Check sheet for the modelled part. Datum: model origin and axes. Units: mm. A direction names the side the tool comes from. Coordinates: 2 decimals unless noted, no trailing zeros. Loops run counter-clockwise (first coordinate to the right, second up) from the corner with the lowest first, then second, coordinate; pieces in that order, holes last. Notation, with made-up numbers: (68, 56) - (77, 56) arc R15 cw to (77, 60) - close; hole circle Ø5 at (86, -19.5). An arc over 180 degrees is marked (long way). Use a Markdown table: item, result. Add a question column.
1) Go/stop test with flat-tipped pins: P1, Ø3, axis at x = -3, y = 2.5, coming from the +Z side; P2, Ø2, axis at x = -2, y = 2, coming from the -Z side (3 decimals); P3, Ø3, axis at x = 4.5, y = -1, coming from the +Z side. Record where each tip stops, or that it passes through.
2) Sectioned sample at C-C, the plane y = 1.5. Enter the section's corners in (x, z) (3 decimals), then the cut area to 4 significant figures.
3) Sectioned sample at B-B, the plane z = -11. Enter the section's corners in (x, y) (3 decimals), then the cut area to 4 significant figures.
4) Tool access check on faces 1 (the cylindrical face through (0.7, 5.76, -45.82)), 2 (the flat face through (0, 2, -12.5)), 3 (the flat face through (0, 4.15, -36)). Record the directions out of +Z, -Z, +X, -X, +Y, -Y that give a thin tool (end or side, any length) a straight path to the whole face; none if there is none.
5) Sectioned sample at A-A, the plane y = 6.5. Enter the section's corners in (x, z) (3 decimals).
6) Draft check along X on faces 4 (the cylindrical face through (-0.348, 6.149, -13.615)), 5 (the cylindrical face through (-3.905, -1.565, -0.867)), 6 (the cylindrical face through (4.946, -1.565, 4.289)). Enter one of: pulls with the +X half, pulls with the -X half, needs draft (parallel to the pull), parting line crosses it, or undercut.
7) Thickness scan on line 1 (Y direction, x = 1, z = -17.5) (3 decimals); line 2 (Z direction, x = -1.5, y = 2.5) (3 decimals); line 3 (Z direction, x = 0.5, y = 7). Record the ranges inside material, lowest first.
from build123d import *

# Parameters (mm, degrees)
SKETCH1_R                    = 4
BASE_FLANGE1_DEPTH           = 3.175
EDGE_FLANGE1_STRIP_W         = 14.1732
EDGE_FLANGE1_STRIP_H         = 3.175
EDGE_FLANGE1_STRIP_CUT_DEPTH = 14
EDGE_FLANGE1_DEPTH           = 14
EDGE_FLANGE2_STRIP_W         = 14.1732
EDGE_FLANGE2_STRIP_H         = 3.175
EDGE_FLANGE2_STRIP_CUT_DEPTH = 14
EDGE_FLANGE2_DEPTH           = 14
SKETCH17_R                   = 3.175
CUT_EXTRUDE1_DEPTH           = 3.175


# Sheet-metal steps are written as plain solids
with BuildPart() as part:
    # Sketch1 → Base-Flange1 (new body)
    with BuildSketch(Plane(origin=(0, 0, 0), x_dir=(1, 0, 0), z_dir=(0, 1, 0))):
        with BuildLine():
            Line((6.750002463, 0), (6.750002463, 12.5))
            Line((6.750002463, 12.5), (-7.249997537, 12.5))
            Line((-7.249997537, 12.5), (-7.249997537, 0))
            ThreePointArc((-7.249997537, 0), (-5.492638224, -4.242640687), (-1.249997537, -6))
            Line((-1.249997537, -6), (0.750002463, -6))
            ThreePointArc((0.750002463, -6), (4.99264315, -4.242640687), (6.750002463, 0))
        make_face()
        with Locations(Location((0, 0, 0), (0, 0, 270))):
            Circle(SKETCH1_R, mode=Mode.SUBTRACT)
    extrude(amount=-BASE_FLANGE1_DEPTH)

    # Edge-Flange1 strip (across the edge) → Edge-Flange1 strip cut (cut)
    with BuildSketch(Plane(origin=(6.750002463, 0, -12.5), x_dir=(0, 0, 1), z_dir=(-1, 0, 0))):
        with Locations((-6.35, -1.5875)):
            Rectangle(EDGE_FLANGE1_STRIP_W, EDGE_FLANGE1_STRIP_H)
    extrude(amount=EDGE_FLANGE1_STRIP_CUT_DEPTH, mode=Mode.SUBTRACT)

    # Edge-Flange1 section (across the edge) → Edge-Flange1 (add)
    with BuildSketch(Plane(origin=(6.750002463, 0, -12.5), x_dir=(0, 0, 1), z_dir=(-1, 0, 0))):
        with BuildLine():
            Line((-3.175, 0.7366), (-3.175, 7.324994814))
            Line((-3.175, 7.324994814), (0, 7.324994814))
            Line((0, 7.324994814), (0, 0.7366))
            ThreePointArc((0, 0.7366), (0.215745145, 0.215745145), (0.7366, 0))
            Line((0.7366, 0), (0.7366, -3.175))
            ThreePointArc((0.7366, -3.175), (-2.029318885, -2.029318885), (-3.175, 0.7366))
        make_face()
    extrude(amount=EDGE_FLANGE1_DEPTH)

    # Edge-Flange2 strip (across the edge) → Edge-Flange2 strip cut (cut)
    with BuildSketch(Plane(origin=(-7.249997537, 7.324994814, -15.675), x_dir=(0, -1, 0), z_dir=(1, 0, 0))):
        with Locations((-3.175, -1.5875)):
            Rectangle(EDGE_FLANGE2_STRIP_W, EDGE_FLANGE2_STRIP_H)
    extrude(amount=EDGE_FLANGE2_STRIP_CUT_DEPTH, mode=Mode.SUBTRACT)

    # Edge-Flange2 section (across the edge) → Edge-Flange2 (add)
    with BuildSketch(Plane(origin=(-7.249997537, 7.324994814, -15.675), x_dir=(0, -1, 0), z_dir=(1, 0, 0))):
        with BuildLine():
            Line((0, 0.7366), (0, 40.175004419))
            Line((0, 40.175004419), (3.175, 40.175004419))
            Line((3.175, 40.175004419), (3.175, 0.7366))
            ThreePointArc((3.175, 0.7366), (3.390745145, 0.215745145), (3.9116, 0))
            Line((3.9116, 0), (3.9116, -3.175))
            ThreePointArc((3.9116, -3.175), (1.145681115, -2.029318885), (0, 0.7366))
        make_face()
    extrude(amount=EDGE_FLANGE2_DEPTH)

    # Sketch17 → Cut-Extrude1 (cut)
    with BuildSketch(Plane(origin=(0, 7.324994814, 0), x_dir=(1, 0, 0), z_dir=(0, 1, 0))):
        with BuildLine():
            ThreePointArc((-7.249997537, 48.850004419), (-5.199745006, 53.799751887), (-0.249997537, 55.850004419))
            Line((-0.249997537, 55.850004419), (-7.249997537, 55.850004419))
            Line((-7.249997537, 55.850004419), (-7.249997537, 48.850004419))
        make_face()
        with BuildLine():
            ThreePointArc((-0.249997537, 55.850004419), (4.699749931, 53.799751887), (6.750002463, 48.850004419))
            Line((6.750002463, 48.850004419), (6.750002463, 55.850004419))
            Line((6.750002463, 55.850004419), (-0.249997537, 55.850004419))
        make_face()
        with Locations(Location((-0.249997537, 48.850004419, 0), (0, 0, 270))):
            Circle(SKETCH17_R)
    extrude(amount=-CUT_EXTRUDE1_DEPTH, mode=Mode.SUBTRACT)


solid = part.part
Solved:
| question | item | result |
|---|---|---|
| 1 | P1 | stops at z = -12.5 |
| 1 | P2 | stops at z = -15.675 |
| 1 | P3 | stops at z = 5.56 |
| 2 | outline | (-7.25, -15.675) - (6.75, -15.675) - (6.75, -12.5) - (-7.25, -12.5) - close |
| 2 | area | 44.45 mm2 |
| 3 | outline | (-7.25, -3.175) - (6.75, -3.175) - (6.75, 0) - (-7.25, 0) - close |
| 3 | area | 44.45 mm2 |
| 4 | face 1 | +Y, -Y |
| 4 | face 2 | +Z, +X, -X, +Y |
| 4 | face 3 | -Z, +X, -X, -Y |
| 5 | outline | (-7.25, -48.85) arc R7 ccw to (6.75, -48.85) - (6.75, -14.009) - (-7.25, -14.009) - close; hole circle Ø6.35 at (-0.25, -48.85) |
| 6 | face 4 | needs draft |
| 6 | face 5 | undercut |
| 6 | face 6 | pulls with the +X half |
| 7 | line 1 | y = 4.15 to 7.325 |
| 7 | line 2 | z = -15.675 to -12.5 |
| 7 | line 3 | z = -55.81 to -51.94, -45.76 to -14.85 |
